Part model, mm, in its own coordinate system. Face numbers are marked on the shaded views. Round coordinates to 2 decimals unless told otherwise and drop trailing zeros. Loops run counter-clockwise (first coordinate to the right, second up) from the corner with the lowest first, then second, coordinate; pieces in that order, holes last. Notation, with made-up numbers: (41, 44) -> (72, 44) arc R31 cw to (72, 74) -> close; hole circle Ø11 at (41.5, 86). An arc over 180 degrees is marked (long way). Use a Markdown table: item, result. Add a question column.
Item 1: Flat gauge pins, fed straight in: pin 1 (0.7 mm diameter, centred on x = -15, z = -25.5, fed in from +Y); pin 2 (1 mm diameter, centred on x = -13, z = -23.5, fed in from +Y); pin 3 (0.7 mm diameter, centred on x = -7.5, z = -24, fed in from +Y). Where does each tip first touch, or does it go through?
Item 2: Probe line 1 (X direction, y = 11.75, z = -19.05) (3 decimals); line 2 (X direction, y = 11.5, z = -4) (3 decimals); line 3 (Z direction, x = -25.4, y = 5). List the from-to ranges inside material, lowest first. Write a range as [from, to].
Item 3: Cut at A-A, the plane x = -25.4. List the corners of the cut face in (y, z), plus the area to 3 significant figures.
Item 4: Two-plate mould, pull along Z, no slides. Class the marked faces 1, 2 and 3: pulls with the +Z half, pulls with the -Z half, needs draft (parallel to the pull), parting line crosses it, or undercut.
Item 5: Cut at D-D, the plane x = 1.5. List the corners of the cut face in (y, z).
Item 6: Cut at C-C, the plane z = -19.05. State how many separate pieces and enclosed holes the cut face has, plus the area to 3 significant figures.
Item 7: Cut at B-B, the plane y = 2. List the corners of the cut face in (x, z) (3 decimals), plus the area to 3 significant figures.
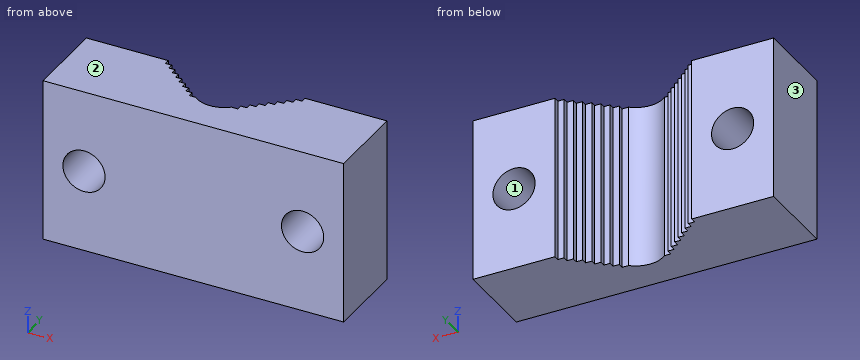
```python
from build123d import *

# Parameters (mm, degrees)
SKETCH1_W               = 69.85
SKETCH1_H               = 19.05
BOSS_EXTRUDE1_DEPTH     = 38.1
CUT_EXTRUDE1_REACH      = 40.1
F_3_8_CLEARANCE_HOLE1_D = 9.8044


with BuildPart() as part:
    # Sketch1 → Boss-Extrude1 (new body)
    with BuildSketch(Plane.XY):
        with Locations((0, 9.525)):
            Rectangle(SKETCH1_W, SKETCH1_H)
    extrude(amount=-BOSS_EXTRUDE1_DEPTH)

    # Sketch2 → Cut-Extrude1 (cut, up to next)
    with BuildSketch(Plane.XY, mode=Mode.PRIVATE) as cut_extrude1_sk1:
        with BuildLine():
            Line((-15.875, 19.05), (0, 19.05))
            Line((0, 19.05), (15.875, 19.05))
            Line((15.875, 19.05), (15.875, 17.78))
            Line((15.875, 17.78), (14.410694861, 17.78))
            Line((14.410694861, 17.78), (14.410694861, 16.51))
            Line((14.410694861, 16.51), (12.946389723, 16.51))
            Line((12.946389723, 16.51), (12.946389723, 15.24))
            Line((12.946389723, 15.24), (11.482084584, 15.24))
            Line((11.482084584, 15.24), (11.482084584, 13.97))
            Line((11.482084584, 13.97), (10.017779445, 13.97))
            Line((10.017779445, 13.97), (10.017779445, 12.7))
            Line((10.017779445, 12.7), (8.553474306, 12.7))
            Line((8.553474306, 12.7), (8.553474306, 11.43))
            Line((8.553474306, 11.43), (7.089169168, 11.43))
            Line((7.089169168, 11.43), (7.089169168, 10.16))
            Line((7.089169168, 10.16), (5.624864029, 10.16))
            Line((5.624864029, 10.16), (5.624864029, 8.89))
            Line((5.624864029, 8.89), (4.16055889, 8.89))
            ThreePointArc((4.16055889, 8.89), (0, 7.337108475), (-4.16055889, 8.89))
            Line((-4.16055889, 8.89), (-5.624864029, 8.89))
            Line((-5.624864029, 8.89), (-5.624864029, 10.16))
            Line((-5.624864029, 10.16), (-7.089169168, 10.16))
            Line((-7.089169168, 10.16), (-7.089169168, 11.43))
            Line((-7.089169168, 11.43), (-8.553474306, 11.43))
            Line((-8.553474306, 11.43), (-8.553474306, 12.7))
            Line((-8.553474306, 12.7), (-10.017779445, 12.7))
            Line((-10.017779445, 12.7), (-10.017779445, 13.97))
            Line((-10.017779445, 13.97), (-11.482084584, 13.97))
            Line((-11.482084584, 13.97), (-11.482084584, 15.24))
            Line((-11.482084584, 15.24), (-12.946389723, 15.24))
            Line((-12.946389723, 15.24), (-12.946389723, 16.51))
            Line((-12.946389723, 16.51), (-14.410694861, 16.51))
            Line((-14.410694861, 16.51), (-14.410694861, 17.78))
            Line((-14.410694861, 17.78), (-15.875, 17.78))
            Line((-15.875, 17.78), (-15.875, 19.05))
        make_face()
    cut_extrude1_tool1 = extrude(cut_extrude1_sk1.sketch, amount=-CUT_EXTRUDE1_REACH, mode=Mode.PRIVATE) & part.part
    add(cut_extrude1_tool1.solids().sort_by_distance((0, 14.620592, 0))[0], mode=Mode.SUBTRACT)

    # 3/8 Clearance Hole1 (through all)
    with Locations(Plane(origin=(0, 19.05, 0), x_dir=(1, 0, 0), z_dir=(0, 1, 0))):
        with Locations((-25.4, 19.05), (25.4, 19.05)):
            Hole(F_3_8_CLEARANCE_HOLE1_D / 2)


solid = part.part
```
A:
| question | item | result |
|---|---|---|
| 1 | pin 1 | stops at y = 17.78 |
| 1 | pin 2 | stops at y = 16.51 |
| 1 | pin 3 | stops at y = 11.43 |
| 2 | line 1 | x = [-34.925, -30.302], [-20.498, -8.553], [8.553, 20.498], [30.302, 34.925] |
| 2 | line 2 | x = [-34.925, -8.553], [8.553, 34.925] |
| 2 | line 3 | z = [-38.1, -23.95], [-14.15, 0] |
| 3 | outline | (0, -38.1) -> (19.05, -38.1) -> (19.05, -23.95) -> (0, -23.95) -> close; (0, -14.15) -> (19.05, -14.15) -> (19.05, 0) -> (0, 0) -> close |
| 3 | area | 539 mm^2 |
| 4 | face 1 | undercut |
| 4 | face 2 | pulls with the +Z half |
| 4 | face 3 | needs draft |
| 5 | outline | (0, -38.1) -> (7.52, -38.1) -> (7.52, 0) -> (0, 0) -> close |
| 6 | separate pieces | 3 |
| 6 | enclosed holes | 0 |
| 6 | area | 730 mm^2 |
| 7 | outline | (-34.925, -38.1) -> (34.925, -38.1) -> (34.925, 0) -> (-34.925, 0) -> close; hole circle Ø9.804 at (-25.4, -19.05); hole circle Ø9.804 at (25.4, -19.05) |
| 7 | area | 2,510 mm^2 |
